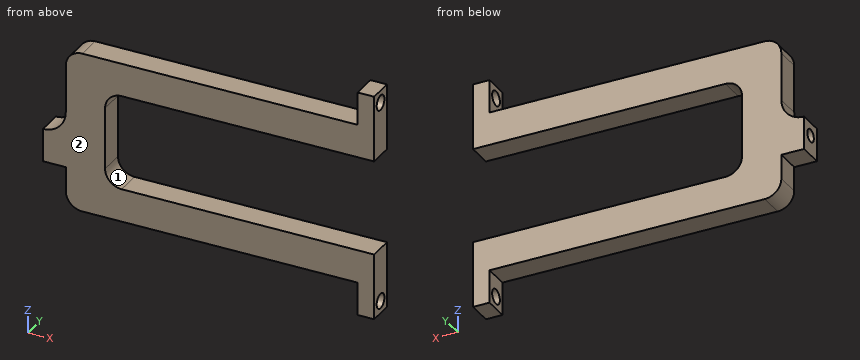
Autodesk Inventor part; units mm, degrees
ref_plane "YZ Plane" through (0, 0, 0) normal (1, 0, 0) x (0, 1, 0)
ref_plane "XZ Plane" through (0, 0, 0) normal (0, 1, 0) x (-1, 0, 0)
ref_plane "XY Plane" through (0, 0, 0) normal (0, 0, 1) x (1, 0, 0)
sketch "Skizze1" plane through (0, 0, 0) normal (0, 1, 0) x (-1, 0, 0)
  line L0 (0, 0) -> (380.5546, 0) construction
  line L1 (20, 97.5) -> (352.5, 97.5)
  line L2 (352.5, -97.5) -> (20, -97.5)
  line L3 (0, 76.1809) -> (0, 137.5)
  line L4 (0, 137.5) -> (20, 137.5)
  line L5 (20, 137.5) -> (20, 97.5)
  line L6 (20, -97.5) -> (20, -137.5)
  line L7 (20, -137.5) -> (0, -137.5)
  line L8 (0, -137.5) -> (0, -73.203)
  line L9 (400, -8.0546) -> (400, -8.0546)
  line L10 (400, -8.0546) -> (400, -48.0546)
  line L11 (400, -48.0546) -> (372.5, -48.0546)
  line L12 (0, 57.5) -> (305, 57.5)
  line L13 (325, 37.5) -> (325, -37.5)
  line L14 (305, -57.5) -> (0, -57.5)
  line L15 (0, -73.203) -> (0, -57.5)
  line L16 (0, 57.5) -> (0, 76.1809)
  line L17 (372.5, 77.5) -> (372.5, 19.4454)
  line L18 (372.5, -48.0546) -> (372.5, -77.5)
  arc A0 (372.5, 19.4454) -> (400, -8.0546) centre (400, 19.4454) ccw
  arc A1 (372.5, 77.5) -> (352.5, 97.5) centre (352.5, 77.5) ccw
  arc A2 (352.5, -97.5) -> (372.5, -77.5) centre (352.5, -77.5) ccw
  arc A3 (325, 37.5) -> (305, 57.5) centre (305, 37.5) ccw
  arc A4 (305, -57.5) -> (325, -37.5) centre (305, -37.5) ccw
  point P0 (372.5, 48.4727)
  dimension "d3" = 57.5
  dimension "d4" = 57.5
  dimension "d7" = 20
  dimension "d8" = 20
  dimension "d11" = 40
  dimension "d12" = 47.5
  dimension "d13" = 27.5
  dimension "d14" = 27.5
  dimension "d18" = 97.5
  dimension "d19" = 97.5
  dimension "d20" = 20
  dimension "d22" = 40
  dimension "d24" = 305
  dimension "d45" = 40
  dimension "d46" = 40
  dimension "d47" = 40
extrude "Extrusion1" add sketch "Skizze1" along normal blind 30
sketch "Skizze2" plane through (-400, 0, -48.0546) normal (-1, 0, 0) x (0, 0, 1)
  line L0 (0, 0) -> (0, 30)
  line L1 (0, 0) -> (40, 0)
  point P0 (48.0546, 0)
  point P1 (24, 15)
  point P2 (0, 15)
  dimension "d34" = 24
hole "Bohrung1" at (-400, 15, -24.0546) direction (1, 0, 0) diameter 15.2937 depth 45
sketch "Skizze3" plane through (-20, 0, 97.5) normal (-1, 0, 0) x (0, 0, 1)
  line L0 (40, 0) -> (40, 30)
  line L1 (-235, 0) -> (-235, 30)
  point P0 (-97.5, 0)
  point P1 (25, 15)
  point P2 (-220, 15)
  point P3 (40, 15)
  point P4 (-235, 15)
  dimension "d43" = 15
  dimension "d44" = 15
hole "Bohrung2" at (-20, 15, 122.5) at (-20, 15, -122.5) direction (1, 0, 0) diameter 18 depth 20
equation "\"d4\" = d3"
equation "\"d8\" = d7"
equation "\"d46\" = d45"
equation "\"d47\" = d22"
properties part number "2" material "Kupfer, Legierung"
Geometry: final body of the model. Coordinates: model frame, mm. Face numbers are marked on the shaded views. A direction names the side the tool comes from. Round coordinates to 2 decimals unless told otherwise and drop trailing zeros. Order: outer loops, then holes, each group sorted by start corner. A loop starts at its lowest first (then second) coordinate and runs counter-clockwise, first axis right, second up. Notation, with made-up numbers: (34, 72) -> (73, 72) arc R20 cw to (73, 78) -> close; hole circle Ø8 at (-19.75, 41.25). An arc over 180 degrees is marked (long way). Use CSV: the item, a comma, the result in double quotes. Start each with the question number.
1) Section C-C (x = -276). Return the cut outline in (y, z).
2) Section B-B (z = -122.5). Return the cut outline in (x, y), and give its area (3 significant figures).
3) Section D-D (z = 4.5). Return the cut outline in (x, y).
4) First-contact query: pin 1 Ø6 at (y, z) = (13, -1) entering from -X; pin 2 Ø14.5 at (y, z) = (11, -56.5) entering from -X; pin 3 Ø2 at (y, z) = (26.5, 16.5) entering from +X; pin 4 Ø11 at (y, z) = (15, -122.5) entering from -X. Flat tips, straight axial feed; report the tip coordinate or a pass-through.
5) Material intervals for line 1 along Z through (x, y) = (-16, 15); line 2 along Y through (x, z) = (-9.25, 122.5); line 3 along Z through (x, y) = (-244, 14.25), sorted ascending. Write a range as from..to.
6) Section A-A (y = 15). State how many separate pieces and enclosed holes the cut face has, and give its area (3 significant figures).
7) Set-up query: the marked faces 1 and 2. Return all of +Z, -Z, +X, -X, +Y, -Y with unobstructed straight access to the full face (end or side cutting, diameter ignored); none if empty.
Returned:
1,outline,"(0, -97.5) -> (30, -97.5) -> (30, -57.5) -> (0, -57.5) -> close; (0, 57.5) -> (30, 57.5) -> (30, 97.5) -> (0, 97.5) -> close"
2,outline,"(-20, 0) -> (0, 0) -> (0, 6) -> (-20, 6) -> close; (-20, 24) -> (0, 24) -> (0, 30) -> (-20, 30) -> close"
2,area,"240 mm²"
3,outline,"(-376.92, 0) -> (-325, 0) -> (-325, 30) -> (-376.92, 30) -> close"
4,pin 1,"stops at x = -385.63"
4,pin 2,"stops at x = -372.5"
4,pin 3,"stops at x = -325"
4,pin 4,"passes through"
5,line 1,"z = -137.5..-131.5, -113.5..-57.5, 57.5..113.5, 131.5..137.5"
5,line 2,"y = 0..6, 24..30"
5,line 3,"z = -97.5..-57.5, 57.5..97.5"
6,separate pieces,"3"
6,enclosed holes,"0"
6,area,"36,700 mm²"
7,face 1,"+X, +Y, -Y"
7,face 2,"+Z, -Z, +X, -X, -Y"
